For this review, use the dimensioned drawing (mm, ordinates from the lowest corner) and the shaded views. Coordinates: 2 decimals unless noted, no trailing zeros. Write each loop counter-clockwise with the first axis right and the second up, starting at its lowest first coordinate (ties: lowest second). Pieces come first, ordered by that corner, then holes. Notation, with made-up numbers: (5, 75.5) - (56, 75.5) arc R14 ccw to (56, 80.5) - close; hole circle Ø11 at (-23.5, -17.5). An arc over 180 degrees is marked (long way). Answer as a JSON object with one key per item and string values.
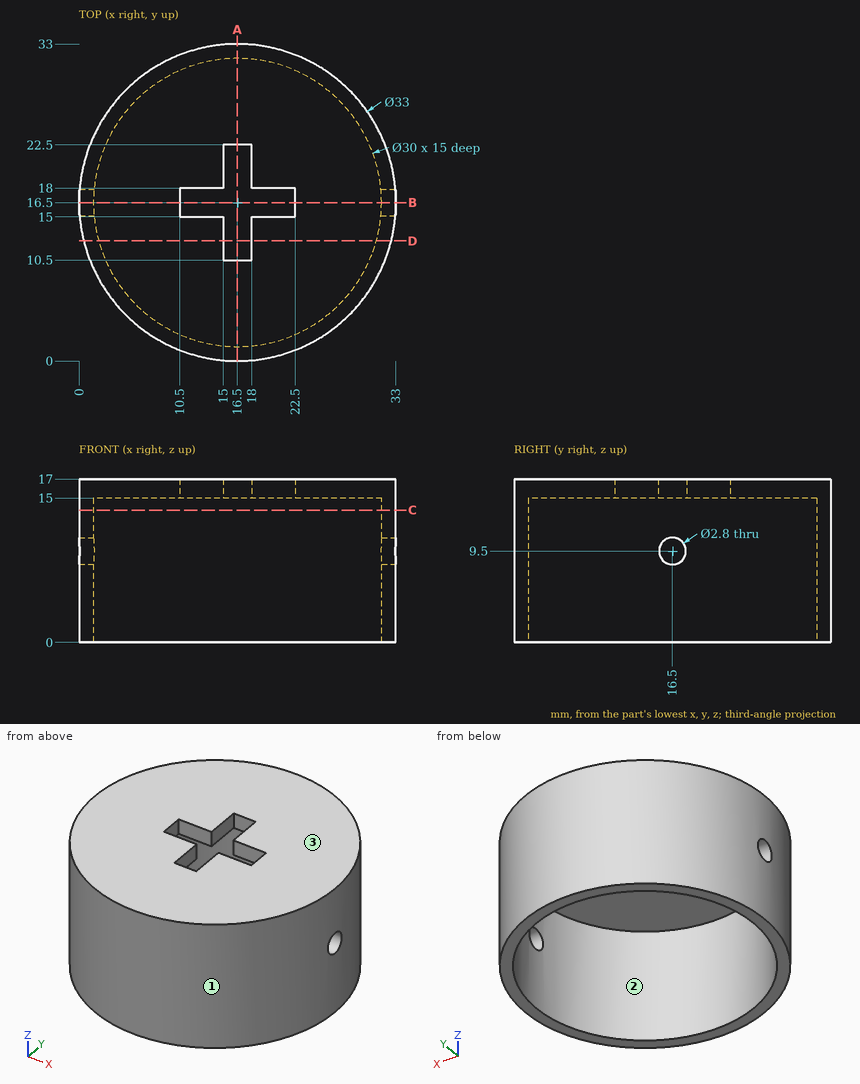
(1) Take a section at B-B, the plane y = 16.5. Write out the cut boundary in (x, z).
Solved:
{"outline": "(0, 0) - (1.5, 0) - (1.5, 8.1) - (0, 8.1) - close; (0, 10.9) - (1.5, 10.9) - (1.5, 15) - (10.5, 15) - (10.5, 17) - (0, 17) - close; (22.5, 15) - (31.5, 15) - (31.5, 10.9) - (33, 10.9) - (33, 17) - (22.5, 17) - close; (31.5, 0) - (33, 0) - (33, 8.1) - (31.5, 8.1) - close"}
(2) Take a section at C-C, the plane z = 13.75. Write out the cut boundary in (x, y), and give its area (3 significant figures).
Solved:
{"outline": "circle Ø33 at (16.5, 16.5); hole circle Ø30 at (16.5, 16.5)", "area": "148 mm^2"}
(3) To check wall thickness, follow line 1 (Y direction, x = 16.5, z = 9); line 2 (Y direction, x = 26.5, z = 7.75); line 3 (X direction, y = 25, z = 8.25). State the ranges of each line that lie inside material, in increasing order. Write a range as from..to.
Solved:
{"line 1": "y = 0..1.5, 31.5..33", "line 2": "y = 3.38..5.32, 27.68..29.62", "line 3": "x = 2.36..4.14, 28.86..30.64"}
(4) The part is to be moulded in two halves that separate along Y. For the marked faces 1, 2 and 3, say which applies: pulls with the +Y half, pulls with the -Y half, needs draft (parallel to the pull), parting line crosses it, or undercut.
Solved:
{"face 1": "parting line crosses it", "face 2": "undercut", "face 3": "needs draft"}
(5) For pin 1 (1 mm diameter, centred on x = 13, z = 16, fed in from +Y) (3 decimals); pin 2 (1.5 mm diameter, centred on y = 19, z = 10, fed in from -X); pin 3 (1.6 mm diameter, centred on x = 20, z = 15.5, fed in from -Y), all flat-tipped, find the tip position at first contact; note any pin that passes through.
Solved:
{"pin 1": "stops at y = 32.725", "pin 2": "stops at x = 0.09", "pin 3": "stops at y = 0.22"}
(6) Take a section at A-A, the plane x = 16.5. Write out the cut boundary in (y, z).
Solved:
{"outline": "(0, 0) - (1.5, 0) - (1.5, 15) - (10.5, 15) - (10.5, 17) - (0, 17) - close; (22.5, 15) - (31.5, 15) - (31.5, 0) - (33, 0) - (33, 17) - (22.5, 17) - close"}
(7) Take a section at D-D, the plane y = 12.5. Write out the cut boundary in (x, z), and give its area (3 significant figures).
Solved:
{"outline": "(0.49, 0) - (2.04, 0) - (2.04, 15) - (15, 15) - (15, 17) - (0.49, 17) - close; (18, 15) - (30.96, 15) - (30.96, 0) - (32.51, 0) - (32.51, 17) - (18, 17) - close", "area": "105 mm^2"}
